```python
from build123d import *

# Parameters (mm, degrees)
SKETCH_1_W           = 98.8
SKETCH_1_H           = 251.6
EXTRUDE_1_DEPTH      = 3
SKETCH_2_W           = 16
SKETCH_2_H           = 25
CUT_EXTRUDE_1_DEPTH  = 271.320180527
CUT_EXTRUDE_2_DEPTH  = 271.320180527
SKETCH_5_R           = 1
CUT_EXTRUDE_3_DEPTH  = 271.320180527
SKETCH_5_3_R         = 1.5
SKETCH_5_3_R_2       = 1
CUT_EXTRUDE_4_DEPTH  = 1.5
SKETCH_6_R           = 1.5
SKETCH_6_R_2         = 1
CUT_EXTRUDE_7_DEPTH  = 1.5
SKETCH_6_2_R         = 1
CUT_EXTRUDE_8_DEPTH  = 271.320180527
SKETCH_7_W           = 8.2
SKETCH_7_H           = 9
CUT_EXTRUDE_9_DEPTH  = 1.5
SKETCH_8_R           = 1
CUT_EXTRUDE_10_DEPTH = 271.320180527
SKETCH_8_3_R         = 1.5
SKETCH_8_3_R_2       = 1
CUT_EXTRUDE_11_DEPTH = 1.5
SKETCH_9_R           = 1
CUT_EXTRUDE_12_DEPTH = 271.320180527
SKETCH_9_3_R         = 1.5
SKETCH_9_3_R_2       = 1
CUT_EXTRUDE_13_DEPTH = 1.5


with BuildPart() as part:
    # 草图1 → 凸台-拉伸1 (new body)
    with BuildSketch(Plane(origin=(0, 0, 0), x_dir=(0, 0, -1), z_dir=(1, 0, 0))):
        with Locations((49.4, -125.8)):
            Rectangle(SKETCH_1_W, SKETCH_1_H)
    extrude(amount=EXTRUDE_1_DEPTH)

    # 草图2 → 切除-拉伸1 (cut, through all)
    with BuildSketch(Plane(origin=(3, 0, 0), x_dir=(0, 0, -1), z_dir=(1, 0, 0))):
        with Locations((8, -51.2)):
            Rectangle(SKETCH_2_W, SKETCH_2_H)
        with Locations((90.8, -51.2)):
            Rectangle(SKETCH_2_W, SKETCH_2_H)
        with Locations((8, -202.3)):
            Rectangle(SKETCH_2_W, SKETCH_2_H)
        with Locations((90.8, -202.3)):
            Rectangle(SKETCH_2_W, SKETCH_2_H)
    extrude(amount=-CUT_EXTRUDE_1_DEPTH, mode=Mode.SUBTRACT)

    # 草图4 → 切除-拉伸2 (cut, through all)
    with BuildSketch(Plane(origin=(3, 0, 0), x_dir=(0, 0, -1), z_dir=(1, 0, 0))):
        Polygon((24.103130316, -62.678318707), (18, -51.2), (24.103130316, -39.721681293), (6.444178459, -30.332250037), (0, -37.242785378), (0, -38.7), (16, -38.7), (16, -63.7), (0, -63.7), (0, -65.157214622), (6.444178459, -72.067749963), align=None)
        Polygon((74.696869684, -39.721681293), (80.8, -51.2), (74.696869684, -62.678318707), (92.355821541, -72.067749963), (98.8, -65.157214622), (98.8, -63.7), (82.8, -63.7), (82.8, -38.7), (98.8, -38.7), (98.8, -37.242785378), (92.355821541, -30.332250037), align=None)
    extrude(amount=-CUT_EXTRUDE_2_DEPTH, mode=Mode.SUBTRACT)

    # 草图5 → 切除-拉伸3 (cut, through all)
    with BuildSketch(Plane.ZY):
        with Locations((-38.45, -51.2)):
            Circle(SKETCH_5_R)
        with Locations((-60.35, -51.2)):
            Circle(SKETCH_5_R)
    extrude(amount=-CUT_EXTRUDE_3_DEPTH, mode=Mode.SUBTRACT)

    # 草图5<3> → 切除-拉伸4 (cut)
    # profile 1 of 2: a face of its own
    with BuildSketch(Plane.ZY):
        with Locations((-38.45, -51.2)):
            Circle(SKETCH_5_3_R)
        with Locations((-38.45, -51.2)):
            Circle(SKETCH_5_3_R_2, mode=Mode.SUBTRACT)
    # profile 2 of 2: a face of its own
    with BuildSketch(Plane.ZY):
        with Locations((-60.35, -51.2)):
            Circle(SKETCH_5_3_R)
        with Locations((-60.35, -51.2)):
            Circle(SKETCH_5_3_R_2, mode=Mode.SUBTRACT)
    extrude(amount=-CUT_EXTRUDE_4_DEPTH, mode=Mode.SUBTRACT)

    # 草图6 → 切除-拉伸7 (cut)
    # profile 1 of 2: a face of its own
    with BuildSketch(Plane.ZY):
        with Locations((-45.65, -88)):
            Circle(SKETCH_6_R)
        with Locations((-45.65, -88)):
            Circle(SKETCH_6_R_2, mode=Mode.SUBTRACT)
    # profile 2 of 2: a face of its own
    with BuildSketch(Plane.ZY):
        with Locations((-53.15, -88)):
            Circle(SKETCH_6_R)
        with Locations((-53.15, -88)):
            Circle(SKETCH_6_R_2, mode=Mode.SUBTRACT)
    extrude(amount=-CUT_EXTRUDE_7_DEPTH, mode=Mode.SUBTRACT)

    # 草图6<2> → 切除-拉伸8 (cut, through all)
    with BuildSketch(Plane.ZY):
        with Locations((-45.65, -88)):
            Circle(SKETCH_6_2_R)
        with Locations((-53.15, -88)):
            Circle(SKETCH_6_2_R)
    extrude(amount=-CUT_EXTRUDE_8_DEPTH, mode=Mode.SUBTRACT)

    # 草图7 → 切除-拉伸9 (cut)
    with BuildSketch(Plane(origin=(3, 0, 0), x_dir=(0, 0, -1), z_dir=(1, 0, 0))):
        with Locations((29.1, -202.3)):
            Rectangle(SKETCH_7_W, SKETCH_7_H)
    extrude(amount=-CUT_EXTRUDE_9_DEPTH, mode=Mode.SUBTRACT)

    # 草图8 → 切除-拉伸10 (cut, through all)
    with BuildSketch(Plane.ZY):
        with Locations((-79.45, -197.6)):
            Circle(SKETCH_8_R)
        with Locations((-79.45, -207)):
            Circle(SKETCH_8_R)
        with Locations((-19.35, -207)):
            Circle(SKETCH_8_R)
        with Locations((-19.35, -197.6)):
            Circle(SKETCH_8_R)
    extrude(amount=-CUT_EXTRUDE_10_DEPTH, mode=Mode.SUBTRACT)

    # 草图8<3> → 切除-拉伸11 (cut)
    # profile 1 of 4: a face of its own
    with BuildSketch(Plane.ZY):
        with Locations((-79.45, -197.6)):
            Circle(SKETCH_8_3_R)
        with Locations((-79.45, -197.6)):
            Circle(SKETCH_8_3_R_2, mode=Mode.SUBTRACT)
    # profile 2 of 4: a face of its own
    with BuildSketch(Plane.ZY):
        with Locations((-79.45, -207)):
            Circle(SKETCH_8_3_R)
        with Locations((-79.45, -207)):
            Circle(SKETCH_8_3_R_2, mode=Mode.SUBTRACT)
    # profile 3 of 4: a face of its own
    with BuildSketch(Plane.ZY):
        with Locations((-19.35, -207)):
            Circle(SKETCH_8_3_R)
        with Locations((-19.35, -207)):
            Circle(SKETCH_8_3_R_2, mode=Mode.SUBTRACT)
    # profile 4 of 4: a face of its own
    with BuildSketch(Plane.ZY):
        with Locations((-19.35, -197.6)):
            Circle(SKETCH_8_3_R)
        with Locations((-19.35, -197.6)):
            Circle(SKETCH_8_3_R_2, mode=Mode.SUBTRACT)
    extrude(amount=-CUT_EXTRUDE_11_DEPTH, mode=Mode.SUBTRACT)

    # 草图9 → 切除-拉伸12 (cut, through all)
    with BuildSketch(Plane.ZY):
        with Locations((-66.1, -189.8)):
            Circle(SKETCH_9_R)
        with Locations((-32.7, -189.8)):
            Circle(SKETCH_9_R)
        with Locations((-66.1, -214.8)):
            Circle(SKETCH_9_R)
        with Locations((-32.7, -214.8)):
            Circle(SKETCH_9_R)
    extrude(amount=-CUT_EXTRUDE_12_DEPTH, mode=Mode.SUBTRACT)

    # 草图9<3> → 切除-拉伸13 (cut)
    # profile 1 of 4: a face of its own
    with BuildSketch(Plane.ZY):
        with Locations((-66.1, -189.8)):
            Circle(SKETCH_9_3_R)
        with Locations((-66.1, -189.8)):
            Circle(SKETCH_9_3_R_2, mode=Mode.SUBTRACT)
    # profile 2 of 4: a face of its own
    with BuildSketch(Plane.ZY):
        with Locations((-32.7, -189.8)):
            Circle(SKETCH_9_3_R)
        with Locations((-32.7, -189.8)):
            Circle(SKETCH_9_3_R_2, mode=Mode.SUBTRACT)
    # profile 3 of 4: a face of its own
    with BuildSketch(Plane.ZY):
        with Locations((-66.1, -214.8)):
            Circle(SKETCH_9_3_R)
        with Locations((-66.1, -214.8)):
            Circle(SKETCH_9_3_R_2, mode=Mode.SUBTRACT)
    # profile 4 of 4: a face of its own
    with BuildSketch(Plane.ZY):
        with Locations((-32.7, -214.8)):
            Circle(SKETCH_9_3_R)
        with Locations((-32.7, -214.8)):
            Circle(SKETCH_9_3_R_2, mode=Mode.SUBTRACT)
    extrude(amount=-CUT_EXTRUDE_13_DEPTH, mode=Mode.SUBTRACT)


solid = part.part
```
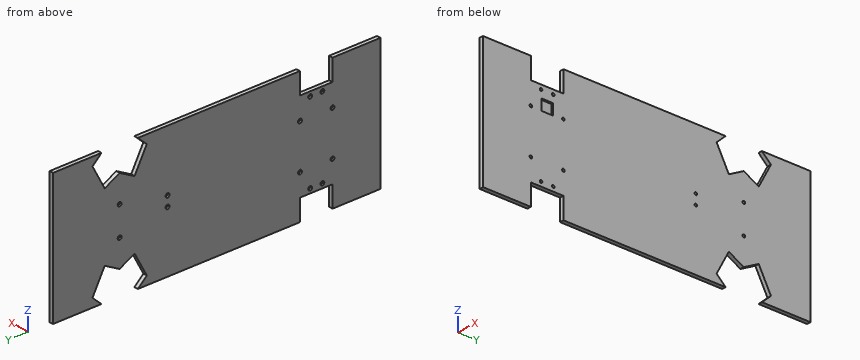
Model file for the job. Use its own axes, mm. Round coordinates to 2 decimals unless told otherwise and drop trailing zeros. Order: outer loops, then holes, each group sorted by start corner. A loop starts at its lowest first (then second) coordinate and runs counter-clockwise, first axis right, second up. Notation, with made-up numbers: (44, 72.5) -> (97, 72.5) arc R25 ccw to (97, 85.5) -> close; hole circle Ø4 at (39.5, 12). An arc over 180 degrees is marked (long way). Use one line per item in the form item = value.
Item 1: Cut at A-A, the plane z = -10.5. Write the cut outline in (x, y).
Returned:
outline = (0, -251.6) -> (3, -251.6) -> (3, -214.8) -> (0, -214.8) -> close; (0, -189.8) -> (3, -189.8) -> (3, -69.91) -> (0, -69.91) -> close; (0, -32.49) -> (3, -32.49) -> (3, 0) -> (0, 0) -> close
Item 2: Drill centre lines: line 1 (Y direction, x = 0.4, z = -32.7); line 2 (Z direction, x = 0.95, y = -197.6); line 3 (Z direction, x = 2.2, y = -66). Where is each one in solid material? Low to high.
Returned:
line_1 = -251.6 to -216.3, -213.3 to -191.3, -188.3 to 0
line_2 = -82.8 to -80.95, -77.95 to -20.85, -17.85 to -16
line_3 = -98.8 to -98.01, -80.94 to -17.86, -0.79 to 0
Item 3: Cut at B-B, the plane x = 0.55. Give the number of separate pieces and of enclosed holes in the cut face, and give its area (3 significant figures).
Returned:
separate_pieces = 1
enclosed_holes = 12
area = 22,500 mm^2
Item 4: Cut at C-C, the plane y = -211. Write the cut outline in (x, z), and give its area (3 significant figures).
Returned:
outline = (0, -82.8) -> (3, -82.8) -> (3, -16) -> (0, -16) -> close
area = 200 mm^2
Item 5: Flat gauge pins, fed straight in: pin 1 Ø0.9 at (y, z) = (-214, -66.5) entering from -X; pin 2 Ø4 at (y, z) = (-200.5, -29.5) entering from +X; pin 3 Ø1.5 at (x, y) = (1, -207.5) entering from -Z. Where does each tip first touch, or does it go through?
Returned:
pin_1 = 1.5
pin_2 = 1.5
pin_3 = -82.8
